Read the model definition and answer for the solid it produces. Units are mm, in the model's axes. A direction names the side the tool comes from. Coordinates: 2 decimals unless noted, no trailing zeros. Order: outer loops, then holes, each group sorted by start corner. A loop starts at its lowest first (then second) coordinate and runs counter-clockwise, first axis right, second up. Notation, with made-up numbers: M 86.25,78 L 93.25,78 A14 ccw 93.25,84 Z; hole C 58,74 d5. An arc over 180 degrees is marked long. Put each result on its own line as item: value.
from build123d import *

# Parameters (mm, degrees)
CUT_EXTRUDE_START   = -3.5
CUT_EXTRUDE_1_DEPTH = 10
SKETCH_3_W          = 4
SKETCH_3_H          = 19.670556204
CUT_EXTRUDE_2_DEPTH = 10
CUT_EXTRUDE_START_2 = -29
SKETCH_4_R          = 4
SKETCH_4_R_2        = 2
CUT_EXTRUDE_3_DEPTH = 29
SKETCH_5_R          = 1
CUT_EXTRUDE_4_DEPTH = 5
SKETCH_6_R          = 2
EXTRUDE_1_DEPTH     = 1
EXTRUDE_START       = -4.5
SKETCH_7_R          = 2.5
SKETCH_7_R_2        = 2
EXTRUDE_2_DEPTH     = 1
SKETCH_8_R          = 1
CUT_EXTRUDE_5_DEPTH = 5
CHAMFER_1_SIZE      = 0.25
CHAMFER_2_SIZE      = 0.25


with BuildPart() as part:
    # 草图1 → 旋转2 (revolve)
    with BuildSketch(Plane.XY, mode=Mode.PRIVATE) as revolve_2_sk:
        Polygon((0, 2), (0, 0), (17, 0), (21, 0), (21, 2), (17, 2), (17, 4), (4, 4), (4, 2), align=None)
    revolve(revolve_2_sk.sketch.rotate(Axis((-16.701754386, 0, 0), (1, 0, 0)), 180), axis=Axis((-16.701754386, 0, 0), (1, 0, 0)))

    # 草图2 → 切除-拉伸1 (cut)
    with BuildSketch(Plane.XY.offset(CUT_EXTRUDE_START)):
        Polygon((12.5, -5.827233832), (12.5, 4), (10.5, 4), (8.5, 4), (8.5, -5.827233832), align=None)
    extrude(amount=-CUT_EXTRUDE_1_DEPTH, mode=Mode.SUBTRACT)

    # 草图3 → 切除-拉伸2 (cut)
    with BuildSketch(Plane(origin=(0, 0, 0), x_dir=(1, 0, 0), z_dir=(0, 1, 0)).offset(CUT_EXTRUDE_START)):
        with Locations((10.5, 3.5)):
            Rectangle(SKETCH_3_W, SKETCH_3_H)
    extrude(amount=-CUT_EXTRUDE_2_DEPTH, mode=Mode.SUBTRACT)

    # 草图4 → 切除-拉伸3 (cut)
    with BuildSketch(Plane(origin=(21, 0, 0), x_dir=(0, 0, -1), z_dir=(1, 0, 0)).offset(CUT_EXTRUDE_START_2)):
        Circle(SKETCH_4_R)
        with Locations(Location((0, 0, 0), (0, 0, 270))):
            Circle(SKETCH_4_R_2, mode=Mode.SUBTRACT)
    extrude(amount=CUT_EXTRUDE_3_DEPTH, mode=Mode.SUBTRACT)

    # 草图5 → 切除-拉伸4 (cut, symmetric)
    with BuildSketch(Plane.XY):
        with Locations((10.5, 0)):
            Circle(SKETCH_5_R)
    extrude(amount=CUT_EXTRUDE_4_DEPTH, both=True, mode=Mode.SUBTRACT)

    # 草图6 → 凸台-拉伸1 (add)
    with BuildSketch(Plane(origin=(21, 0, 0), x_dir=(0, 0, -1), z_dir=(1, 0, 0))):
        with Locations(Location((0, 0, 0), (0, 0, 270))):
            Circle(SKETCH_6_R)
    extrude(amount=EXTRUDE_1_DEPTH)

    # 草图7 → 凸台-拉伸2 (add)
    with BuildSketch(Plane(origin=(22, 0, 0), x_dir=(0, 0, -1), z_dir=(1, 0, 0)).offset(EXTRUDE_START)):
        with Locations(Location((0, 0, 0), (0, 0, 90))):
            Circle(SKETCH_7_R)
        with Locations(Location((0, 0, 0), (0, 0, 270))):
            Circle(SKETCH_7_R_2, mode=Mode.SUBTRACT)
    extrude(amount=EXTRUDE_2_DEPTH)

    # 草图8 → 切除-拉伸5 (cut)
    with BuildSketch(Plane(origin=(22, 0, 0), x_dir=(0, 0, -1), z_dir=(1, 0, 0))):
        with Locations(Location((0, 0, 0), (0, 0, 90))):
            Circle(SKETCH_8_R)
    extrude(amount=-CUT_EXTRUDE_5_DEPTH, mode=Mode.SUBTRACT)

    # 倒角1
    chamfer_1_edges = [part.edges().sort_by_distance(p)[0] for p in [
        (22, 2, 0),
    ]]
    chamfer(chamfer_1_edges, length=CHAMFER_1_SIZE)

    # 倒角2
    chamfer_2_edges = [part.edges().sort_by_distance(p)[0] for p in [
        (0, 2, 0),
    ]]
    chamfer(chamfer_2_edges, length=CHAMFER_2_SIZE)


solid = part.part
Q1. Given pin 1 (3 mm diameter, centred on x = 10.5, y = 0, fed in from +Z); pin 2 (1 mm diameter, centred on x = 7.5, z = 0, fed in from -Y); pin 3 (2 mm diameter, centred on y = 0.5, z = -1.5, fed in from -X); pin 4 (3 mm diameter, centred on x = 10.5, z = 2, fed in from -Y), each flat-ended and moving along its own axis, determine where each tip first touches the part or whether it passes through.
Answers below:
pin 1: stops at z = 2
pin 2: stops at y = -2
pin 3: stops at x = 0
pin 4: stops at y = -1.94
Q2. Find section A-A on y = 0. Write down the section's boundary in (x, z).
Answers below:
outline: M 0,-1.75 L 0.25,-2 L 9.5,-2 L 9.5,2 L 0.25,2 L 0,1.75 Z; M 11.5,-2 L 17.5,-2 L 17.5,-2.5 L 18.5,-2.5 L 18.5,-2 L 21.75,-2 L 22,-1.75 L 22,-1 L 17,-1 L 17,1 L 22,1 L 22,1.75 L 21.75,2 L 18.5,2 L 18.5,2.5 L 17.5,2.5 L 17.5,2 L 11.5,2 Z
Q3. Find section B-B on z = 0. Write down the section's boundary in (x, y), plus the area to 3 significant figures.
Answers below:
outline: M 0,-1.75 L 0.25,-2 L 17.5,-2 L 17.5,-2.5 L 18.5,-2.5 L 18.5,-2 L 21.75,-2 L 22,-1.75 L 22,-1 L 17,-1 L 17,1 L 22,1 L 22,1.75 L 21.75,2 L 18.5,2 L 18.5,2.5 L 17.5,2.5 L 17.5,2 L 0.25,2 L 0,1.75 Z; hole C 10.5,0 d2
area: 75.7 mm^2
Q4. Find section D-D on x = 10.5. Write down the section's boundary in (y, z), plus the area to 3 significant figures.
Answers below:
outline: M -1,-1.73 L -1,1.73 A2 ccw Z; M 1,-1.73 A2 ccw 1,1.73 Z
area: 4.91 mm^2
Q5. Consider line 1 along Z through (x, y) = (20.9, 0); line 2 along X through (y, z) = (0, 0.4); line 3 along X through (y, z) = (0, -1.05). Determine where each line is inside the solid, lowest interval first.
Answers below:
line 1: z = -2 to -1, 1 to 2
line 2: x = 0 to 9.5, 11.5 to 17
line 3: x = 0 to 9.5, 11.5 to 22
Q6. A tool of negligible diameter and unlimited length cuts with its end or side. For faces 1 (the face through (17.5, -1, 2)), 2 (the face through (20, 0, 2)), 3 (the face through (0, 0, 0)), from which of +Z, -Z, +X, -X, +Y, -Y can it reach the whole face along a straight path? Write none if from no direction.
Answers below:
face 1: -X
face 2: +X
face 3: +Z, -Z, -X, +Y, -Y
Q7. For a pull along Y with two mould halves and no side action, classify faces 4 (the face through (17.99, -0.54, -2.44)), 5 (the face through (17, 0, 0)), 6 (the face through (22, -1, 1)) as +Y half, -Y half, draft (parallel to the pull), parting line (faces both ways), or undercut.
Answers below:
face 4: parting line
face 5: undercut
face 6: draft
Q8. Find section C-C on x = 20.5. Write down the section's boundary in (y, z).
Answers below:
outline: C 0,0 d4; hole C 0,0 d2
